from build123d import *

# Parameters (mm, degrees)
EXTRUDE_1_DEPTH      = 83.1
SKETCH_2_W           = 35.4
SKETCH_2_H           = 4.4
SKETCH_2_W_2         = 30.4
CUT_EXTRUDE_1_DEPTH  = 5
SKETCH_3_W           = 35.4
SKETCH_3_H           = 4.4
CUT_EXTRUDE_2_DEPTH  = 5
CUT_EXTRUDE_4_DEPTH  = 21
SKETCH_7_R           = 4.5
CUT_EXTRUDE_5_DEPTH  = 107.120558328
SKETCH_8_R           = 11.1
CUT_EXTRUDE_6_DEPTH  = 7
SKETCH_9_R           = 11.15
CUT_EXTRUDE_7_DEPTH  = 7
CUT_EXTRUDE_8_DEPTH  = 107.120558328
FILLET_1_R           = 10
CUT_EXTRUDE_9_DEPTH  = 18.6
CUT_EXTRUDE_10_DEPTH = 5.42
FILLET_2_R           = 2
FILLET_3_R           = 2
FILLET_4_R           = 4


with BuildPart() as part:
    # Эскиз1 → Бобышка-Вытянуть1 (new body)
    with BuildSketch(Plane(origin=(0, 0, 0), x_dir=(1, 0, 0), z_dir=(0, 1, 0))):
        with BuildLine():
            Line((48.631682576, -27.49140627), (48.632387335, -27.491404976))
            ThreePointArc((48.632387335, -27.491404976), (76.382325871, 0.258533559), (48.632387335, 28.008472095))
            Line((48.632387335, 28.008472095), (-81.367612665, 28.008472095))
            Line((-81.367612665, 28.008472095), (-81.367612665, -27.730072458))
            Line((-81.367612665, -27.730072458), (48.631682576, -27.49140627))
        make_face()
    extrude(amount=EXTRUDE_1_DEPTH)

    # Эскиз2 → Вырез-Вытянуть1 (cut)
    with BuildSketch(Plane(origin=(0, 0, 0), x_dir=(-1, 0, 0), z_dir=(0, -1, 0))):
        with Locations((8.387612665, -21.628577297)):
            Rectangle(SKETCH_2_W, SKETCH_2_H)
        with Locations((45.887612665, 22.008472095)):
            Rectangle(SKETCH_2_W_2, SKETCH_2_H)
        with Locations((0.287612665, 22.008472095)):
            Rectangle(SKETCH_2_W_2, SKETCH_2_H)
    extrude(amount=-CUT_EXTRUDE_1_DEPTH, mode=Mode.SUBTRACT)

    # Эскиз3 → Вырез-Вытянуть2 (cut)
    with BuildSketch(Plane(origin=(0, 83.1, 0), x_dir=(1, 0, 0), z_dir=(0, 1, 0))):
        with Locations((-4.787612665, -24.021972088)):
            Rectangle(SKETCH_3_W, SKETCH_3_H)
    extrude(amount=-CUT_EXTRUDE_2_DEPTH, mode=Mode.SUBTRACT)

    # Эскиз6 → Вырез-Вытянуть4 (cut)
    with BuildSketch(Plane(origin=(0, 83.1, 0), x_dir=(1, 0, 0), z_dir=(0, 1, 0))):
        with BuildLine():
            Line((-38.710860793, -19.821972088), (16.267507788, -19.821972088))
            Line((16.267507788, -19.821972088), (16.267507788, -27.550823779))
            Line((16.267507788, -27.550823779), (37.284075999, -27.512239383))
            ThreePointArc((37.284075999, -27.512239383), (78.632374752, 0.286010542), (37.233224591, 28.008472095))
            Line((37.233224591, 28.008472095), (-1.367612665, 28.008472095))
            Line((-1.367612665, 28.008472095), (-1.367612665, 20.408472095))
            Line((-1.367612665, 20.408472095), (-67.700309337, 20.408472095))
            Line((-67.700309337, 20.408472095), (-73.189452249, 28.008472095))
            Line((-73.189452249, 28.008472095), (-81.367612665, 28.008472095))
            Line((-81.367612665, 28.008472095), (-81.367612665, -27.730072458))
            Line((-81.367612665, -27.730072458), (-32.996113938, -27.641267044))
            Line((-32.996113938, -27.641267044), (-38.710860793, -19.821972088))
        make_face()
    extrude(amount=-CUT_EXTRUDE_4_DEPTH, mode=Mode.SUBTRACT)

    # Эскиз7 → Вырез-Вытянуть5 (cut, through all)
    with BuildSketch(Plane(origin=(0, 62.1, 0), x_dir=(1, 0, 0), z_dir=(0, 1, 0))):
        with Locations(Location((48.632387335, 0.258533559, 0), (0, 0, 270))):
            Circle(SKETCH_7_R)
    extrude(amount=-CUT_EXTRUDE_5_DEPTH, mode=Mode.SUBTRACT)

    # Эскиз8 → Вырез-Вытянуть6 (cut)
    with BuildSketch(Plane(origin=(0, 62.1, 0), x_dir=(1, 0, 0), z_dir=(0, 1, 0))):
        with Locations(Location((48.632387335, 0.258533559, 0), (0, 0, 270))):
            Circle(SKETCH_8_R)
    extrude(amount=-CUT_EXTRUDE_6_DEPTH, mode=Mode.SUBTRACT)

    # Эскиз9 → Вырез-Вытянуть7 (cut)
    with BuildSketch(Plane.XZ):
        with Locations(Location((48.632387335, -0.258533559, 0), (0, 0, 270))):
            Circle(SKETCH_9_R)
    extrude(amount=-CUT_EXTRUDE_7_DEPTH, mode=Mode.SUBTRACT)

    # Эскиз10 → Вырез-Вытянуть8 (cut, through all)
    with BuildSketch(Plane(origin=(0, 62.1, 0), x_dir=(1, 0, 0), z_dir=(0, 1, 0))):
        Polygon((-73.189452249, 28.008472095), (-81.367612665, 28.008472095), (-81.367612665, -27.730072458), (-32.996113938, -27.641267044), align=None)
    extrude(amount=-CUT_EXTRUDE_8_DEPTH, mode=Mode.SUBTRACT)

    # Скругление1
    # the kernel refuses this fillet: 10 mm, written as the material it takes off along each edge
    with BuildSketch(Plane(origin=(-1.367612665, 107.369322199, -28.008472095), x_dir=(0, 0, 1), z_dir=(0, -1, 0))) as fillet_1_piece_1:
        with BuildLine():
            CenterArc((10, 9.70772888), FILLET_1_R, 180, 76.113459637)
            Line((0, 9.70772888), (-0.2, 9.70772888))
            Line((-0.2, 9.70772888), (-0.2, 0))
            Line((-0.2, 0), (0, -0.2))
            ThreePointArc((0, -0.2), (3.8, -0.2), (7.552, -0.194154578))
            Line((7.552, -0.194154578), (7.6, 0))
        make_face()
    extrude(amount=45.269322199, mode=Mode.SUBTRACT)

    # Эскиз11 → Вырез-Вытянуть9 (cut)
    with BuildSketch(Plane(origin=(0, 62.1, 0), x_dir=(1, 0, 0), z_dir=(0, 1, 0))):
        Polygon((-35.9280852, 0.295824639), (-32.155315119, -6.243954097), (-24.605315558, -6.246528733), (-20.828086078, 0.290675368), (-24.600856158, 6.830454104), (-32.150855719, 6.833028739), align=None)
    extrude(amount=-CUT_EXTRUDE_9_DEPTH, mode=Mode.SUBTRACT)

    # Эскиз12 → Вырез-Вытянуть10 (cut)
    with BuildSketch(Plane(origin=(0, 62.1, 0), x_dir=(1, 0, 0), z_dir=(0, 1, 0))):
        Polygon((-1.367612665, 20.408472095), (18.632387335, -19.821972088), (-38.710860793, -19.821972088), (-67.700309337, 20.408472095), align=None)
    extrude(amount=-CUT_EXTRUDE_10_DEPTH, mode=Mode.SUBTRACT)

    # Скругление2
    fillet_2_edges = [part.edges().sort_by_distance(p)[0] for p in [
        (18.632387335, 59.39, 19.821972088),
    ]]
    fillet(fillet_2_edges, radius=FILLET_2_R)

    # Скругление3
    # the kernel refuses this fillet: 2 mm, written as the material it takes off along each edge
    with BuildSketch(Plane(origin=(16.267507788, 88.589321146, 19.62624363), x_dir=(-0.9952454215977946, 0, 0.09739892601373129), z_dir=(0, -1, 0))) as fillet_3_piece_1:
        with BuildLine():
            CenterArc((2.204352437, -1.990490843), FILLET_3_R, 95.589408628, 90)
            Line((0.213861594, -2.185288695), (0.014812509, -2.20476848))
            Line((0.014812509, -2.20476848), (-0.199049084, -0.019479785))
            Line((-0.199049084, -0.019479785), (0.068306766, 0.187973896))
            ThreePointArc((0.068306766, 0.187973896), (0.858385725, 0.088297205), (1.9900748, 0.199049084))
            Line((1.9900748, 0.199049084), (2.009554585, 0))
        make_face()
    extrude(amount=26.489321146, mode=Mode.SUBTRACT)

    # Скругление4
    fillet_4_edges = [part.edges().sort_by_distance(p)[0] for p in [
        (16.267507788, 72.6, 27.550823779),
    ]]
    fillet(fillet_4_edges, radius=FILLET_4_R)


solid = part.part
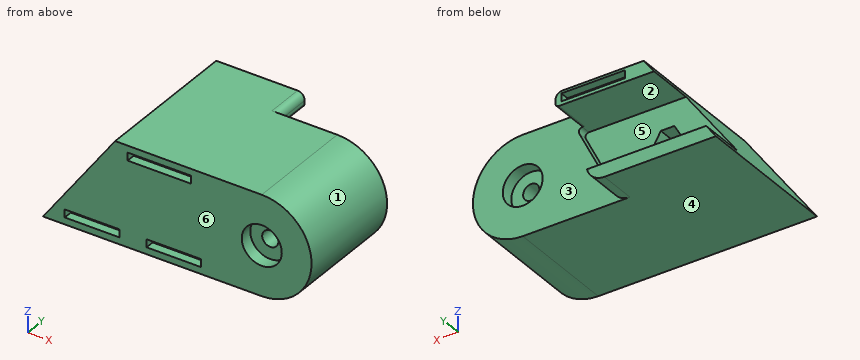
Could you check a few things on this model? Use its own coordinates, in mm. Face numbers are marked on the shaded views. A direction names the side the tool comes from. Give positions to 0.01 mm unless a question says otherwise; leave off trailing zeros. Loops run counter-clockwise (first coordinate to the right, second up) from the corner with the lowest first, then second, coordinate; pieces in that order, holes last. Notation, with made-up numbers: (-7.75, 43.5) -> (41.25, 43.5) arc R17 ccw to (41.25, 60.5) -> close; hole circle Ø6 at (-35.5, 44). An arc over 180 degrees is marked (long way). Answer as CSV lines item,"result". Start each with the question number.
(1) We'd pull the mould along Z, two halves only. Please class the marked faces 1, 2, 3 and 4: released by +Z, released by -Z, zero draft, split by the parting line, or undercut.
(2) If we section it at C-C on z = 2: Write out the boundary of the cut face in (x, y), then the cut area to 3 significant figures.
(3) Which directions (+Z, -Z, +X, -X, +Y, -Y) give clear straight access to the entire face, cutting with the end or side of a thin tool? Please do the marked faces 5 and 6.
(4) If we section it at A-A on y = 64: Write out the boundary of the cut face in (x, z).
(5) I need wall thicknesses on probe 1 along Z at (x, y) = (-15, 57); probe 2 along Y at (x, z) = (10.5, 1.5); probe 3 along Y at (x, z) = (-44, -0.5). Which ranges of each line are inside material? Lowest first, please.
(6) If we section it at D-D on x = 4.5: Write out the boundary of the cut face in (y, z), then the cut area to 3 significant figures.
(7) I'm going to push flat-ended pins straight in: pin 1 Ø4 at (x, z) = (28.5, -14.5) entering from +Y; pin 2 Ø4 at (x, y) = (-9.5, 80.5) entering from +Z; pin 3 Ø1.4 at (y, z) = (77.5, 22.5) entering from +X; pin 4 Ø7 at (x, z) = (48.63, -0.26) entering from -Y. Where does each tip first touch, or does it pass through?
Computed:
1,face 1,"split by the parting line"
1,face 2,"undercut"
1,face 3,"zero draft"
1,face 4,"released by -Z"
2,outline,"(-51.52, 0) -> (37.71, 0) -> (37.71, 7) -> (44.74, 7) -> (44.74, 55.1) -> (37.76, 55.1) -> (37.76, 62.1) -> (9.77, 62.1) -> (9.77, 56.68) -> (-22.15, 56.68) -> (-22.15, 43.5) -> (-34.6, 43.5) -> (-34.6, 56.68) -> (-51.52, 56.68) -> close; (52.52, 7) -> (59.55, 7) -> (59.55, 0) -> (76.29, 0) -> (76.29, 62.1) -> (59.5, 62.1) -> (59.5, 55.1) -> (52.52, 55.1) -> close"
2,area,"6,760 mm2"
3,face 5,"-X, +Y"
3,face 6,"+Z, -Z, +X, -X, -Y"
4,outline,"(-73.19, -28.01) -> (-11.08, -28.01) arc R10 ccw to (-1.37, -20.41) -> (-67.7, -20.41) -> close; (-38.71, 19.82) -> (14.27, 19.82) arc R2 ccw to (16.27, 21.82) -> (16.27, 23.56) arc R4 ccw to (12.27, 27.56) -> (-33, 27.64) -> close"
5,probe 1,"z = -28.01 to -20.41, 19.82 to 27.61"
5,probe 2,"y = 0 to 62.1"
5,probe 3,"y = 0 to 56.68"
6,outline,"(0, -28.01) -> (62.1, -28.01) -> (62.1, -8.61) -> (56.68, -8.61) -> (56.68, 19.82) -> (83.1, 19.82) -> (83.1, 21.82) -> (78.1, 21.82) -> (78.1, 26.22) -> (83.1, 26.22) -> (83.1, 27.57) -> (0, 27.57) -> (0, 23.83) -> (5, 23.83) -> (5, 19.43) -> (0, 19.43) -> (0, -19.81) -> (5, -19.81) -> (5, -24.21) -> (0, -24.21) -> close"
6,area,"3,390 mm2"
7,pin 1,"stops at y = 62.1"
7,pin 2,"stops at z = 27.6"
7,pin 3,"stops at x = 16.27"
7,pin 4,"passes through"
